Work out the finished part from the listing and answer in its coordinate system (mm). Round coordinates to 2 decimals unless told otherwise and drop trailing zeros. Order: outer loops, then holes, each group sorted by start corner. A loop starts at its lowest first (then second) coordinate and runs counter-clockwise, first axis right, second up. Notation, with made-up numbers: (-39, 84.25) - (9, 84.25) arc R4 cw to (9, 90.25) - close; hole circle Ø11 at (-18, -28). An arc over 180 degrees is marked (long way). Put each result on its own line as item: value.
```python
from build123d import *

# Parameters (mm, degrees)
BOSS_EXTRUDE1_DEPTH = 225.79


with BuildPart() as part:
    # Sketch3 → Boss-Extrude1 (new, symmetric)
    with BuildSketch(Plane.XY):
        with BuildLine():
            Line((0, 1.948577375), (0, -0.29197505))
            ThreePointArc((0, -0.29197505), (-0.523261774, -1.555240722), (-1.786527446, -2.078502496))
            ThreePointArc((-1.786527446, -2.078502496), (0, -5.335508002), (-1.348017062, -8.797099424))
            ThreePointArc((-1.348017062, -8.797099424), (-1.44249717, -9.451284226), (-0.829990586, -9.699719191))
            ThreePointArc((-0.829990586, -9.699719191), (1.051740503, -8.676690662), (2.322485679, -6.952536967))
            ThreePointArc((2.322485679, -6.952536967), (2.381708142, -6.755524983), (2.539743588, -6.623821455))
            Line((2.539743588, -6.623821455), (5.300722676, -5.447520291))
            ThreePointArc((5.300722676, -5.447520291), (5.596816097, -4.778241367), (4.949120021, -4.437513638))
            Line((4.949120021, -4.437513638), (2.774145358, -5.033000346))
            ThreePointArc((2.774145358, -5.033000346), (2.463049453, -4.972438368), (2.322485679, -4.68837809))
            Line((2.322485679, -4.68837809), (2.322485679, -1.81903037))
            ThreePointArc((2.322485679, -1.81903037), (2.381708142, -1.622018386), (2.539743588, -1.490314858))
            Line((2.539743588, -1.490314858), (5.300722676, -0.314013694))
            ThreePointArc((5.300722676, -0.314013694), (5.596816097, 0.35526523), (4.949120021, 0.695992958))
            Line((4.949120021, 0.695992958), (2.774145358, 0.10050625))
            ThreePointArc((2.774145358, 0.10050625), (2.463049453, 0.161068229), (2.322485679, 0.445128506))
            Line((2.322485679, 0.445128506), (2.322485679, 2.352673629))
            ThreePointArc((2.322485679, 2.352673629), (3.408861985, 5.798219074), (6.275053034, 7.997524819))
            Line((6.275053034, 7.997524819), (8.06755911, 8.649943675))
            ThreePointArc((8.06755911, 8.649943675), (8.387886595, 9.336888184), (7.700942086, 9.65721567))
            Line((7.700942086, 9.65721567), (-1.504292096, 6.306784428))
            ThreePointArc((-1.504292096, 6.306784428), (-2.356701332, 5.652707816), (-2.679791168, 4.627997771))
            Line((-2.679791168, 4.627997771), (-2.679791168, 3.73510482))
            Line((-2.679791168, 3.73510482), (-1.786527446, 3.73510482))
            ThreePointArc((-1.786527446, 3.73510482), (-0.523261774, 3.211843046), (0, 1.948577375))
        make_face()
    extrude(amount=BOSS_EXTRUDE1_DEPTH, both=True)


solid = part.part
```
1) Given pin 1 Ø5 at (y, z) = (-3.5, 109) entering from +X; pin 2 Ø2.5 at (y, z) = (-2.5, 20.5) entering from +X; pin 3 Ø4 at (x, z) = (0, 179) entering from +Y, each flat-ended and moving along its own axis, determine where each tip first touches the part or whether it passes through.
Findings below:
pin 1: stops at x = 5.63
pin 2: stops at x = 3.1
pin 3: stops at y = 7.58
2) Straight lines are drawn through the part: L1, parallel to Y at x = 4, z = -162.5; L2, parallel to Y at x = -0.75, z = 79; L3, parallel to X at y = 4, z = -169. For each, find the intervals that lie inside material, in ascending order. Write a range as from..to.
Findings below:
L1: y = -6..-4.7, -0.87..0.44, 6.52..8.31
L2: y = -9.68..-8.09, -3.15..-1.75, 3.4..6.58
L3: x = -2.68..2.55
3) A cutting plane is placed at A-A on z = -98.5. Write down the section's boundary in (x, y).
Findings below:
outline: (-2.68, 3.74) - (-1.79, 3.74) arc R1.79 cw to (0, 1.95) - (0, -0.29) arc R1.79 cw to (-1.79, -2.08) arc R4.39 cw to (-1.35, -8.8) arc R0.54 ccw to (-0.83, -9.7) arc R4.93 ccw to (2.32, -6.95) arc R0.36 cw to (2.54, -6.62) - (5.3, -5.45) arc R0.54 ccw to (4.95, -4.44) - (2.77, -5.03) arc R0.36 cw to (2.32, -4.69) - (2.32, -1.82) arc R0.36 cw to (2.54, -1.49) - (5.3, -0.31) arc R0.54 ccw to (4.95, 0.7) - (2.77, 0.1) arc R0.36 cw to (2.32, 0.45) - (2.32, 2.35) arc R6.01 cw to (6.28, 8) - (8.07, 8.65) arc R0.54 ccw to (7.7, 9.66) - (-1.5, 6.31) arc R1.79 ccw to (-2.68, 4.63) - close
